from build123d import *

# Parameters (mm, degrees)
EXTRUDE_1_DEPTH     = 10
SKETCH_2_R          = 2.25
CUT_EXTRUDE_1_DEPTH = 10
SKETCH_3_R          = 2.75
CUT_EXTRUDE_2_DEPTH = 10


with BuildPart() as part:
    # 草图1 → 凸台-拉伸1 (new body)
    with BuildSketch(Plane(origin=(0, 0, 0), x_dir=(0, 0, -1), z_dir=(1, 0, 0))):
        Polygon((-150, -110), (-150, 110), (-60, 150), (60, 150), (150, 110), (150, -110), (60, -150), (-60, -150), align=None)
    extrude(amount=EXTRUDE_1_DEPTH)

    # 草图2 → 切除-拉伸1 (cut)
    with BuildSketch(Plane(origin=(10, 0, 0), x_dir=(0, 0, -1), z_dir=(1, 0, 0))):
        with Locations((92, 30)):
            Circle(SKETCH_2_R)
        with Locations((92, -30)):
            Circle(SKETCH_2_R)
        with Locations((100, 65)):
            Circle(SKETCH_2_R)
        with Locations((100, -65)):
            Circle(SKETCH_2_R)
        with Locations(Location((-100, -65, 0), (0, 0, 180))):
            Circle(SKETCH_2_R)
        with Locations(Location((-100, 65, 0), (0, 0, 180))):
            Circle(SKETCH_2_R)
        with Locations(Location((-92, -30, 0), (0, 0, 180))):
            Circle(SKETCH_2_R)
        with Locations(Location((-92, 30, 0), (0, 0, 180))):
            Circle(SKETCH_2_R)
    extrude(amount=-CUT_EXTRUDE_1_DEPTH, mode=Mode.SUBTRACT)

    # 草图3 → 切除-拉伸2 (cut)
    with BuildSketch(Plane(origin=(10, 0, 0), x_dir=(0, 0, -1), z_dir=(1, 0, 0))):
        with Locations((-90.5, 90.5)):
            Circle(SKETCH_3_R)
        with Locations((90.5, 90.5)):
            Circle(SKETCH_3_R)
        with Locations((-90.5, -90.5)):
            Circle(SKETCH_3_R)
        with Locations((90.5, -90.5)):
            Circle(SKETCH_3_R)
    extrude(amount=-CUT_EXTRUDE_2_DEPTH, mode=Mode.SUBTRACT)


solid = part.part
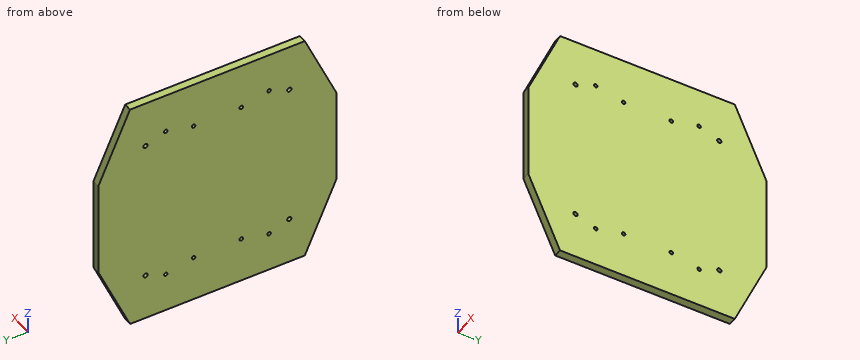
Verification items for the finished model (mm, model axes). Give positions to 0.01 mm unless a question says otherwise; leave off trailing zeros. Loops run counter-clockwise (first coordinate to the right, second up) from the corner with the lowest first, then second, coordinate; pieces in that order, holes last. Notation, with made-up numbers: (1.25, 48) - (39.25, 48) arc R9 ccw to (39.25, 61) - close; hole circle Ø11 at (-32, 30). An arc over 180 degrees is marked (long way). Write each question's results on one line, items separated by ' | '.
1) Sectioned sample at C-C on z = 72.5. Record the boundary of the cut face in (x, y), plus the area to 3 significant figures.
Solution:
outline: (0, -144.44) - (10, -144.44) - (10, 144.44) - (0, 144.44) - close | area: 2,890 mm2
2) Sectioned sample at A-A on x = 3.25. Count the separate pieces of the cut face and the enclosed holes in it, plus the area to 3 significant figures.
Solution:
separate pieces: 1 | enclosed holes: 12 | area: 82,600 mm2
3) Material ranges on L1, parallel to Y at x = 5, z = 100; L2, parallel to Y at x = 6, z = 90.5; L3, parallel to Z at x = 9, y = -32, recorded low to high. Write a range as from..to.
Solution:
L1: -132.22..-67.25, -62.75..62.75, 67.25..132.22 | L2: -136.44..-93.25, -87.75..-31.68, -28.32..28.32, 31.68..87.75, 93.25..136.44 | L3: -150..-93.03, -90.97..90.97, 93.03..150
4) Sectioned sample at B-B on z = -114. Record the boundary of the cut face in (x, y), plus the area to 3 significant figures.
Solution:
outline: (0, -126) - (10, -126) - (10, 126) - (0, 126) - close | area: 2,520 mm2
5) Depth check by flat-ended pin: P1, Ø7, axis at y = 30, z = -92, coming from the -X side. Enter the tip coordinate at first touch or a pass-through.
Solution:
P1: x = 0
